The listing builds one solid part. Answer for the finished solid, in the listing's coordinates (mm). Give positions to 0.01 mm unless a question says otherwise; leave off trailing zeros. Order: outer loops, then holes, each group sorted by start corner. A loop starts at its lowest first (then second) coordinate and runs counter-clockwise, first axis right, second up. Notation, with made-up numbers: (63.25, 51) - (88.25, 51) arc R15 ccw to (88.25, 76) - close; hole circle Ø5 at (-35.75, -35). An arc over 180 degrees is marked (long way). Use CSV: the item, a comma, the result in double quotes.
```python
from build123d import *

# Parameters (mm, degrees)
F0_R     = 7
F0_R_2   = 1.55
F1_DEPTH = 7
F2_R     = 1
F3_R     = 4
F4_DEPTH = 3


with BuildPart() as f1:
    # F0 (on Front) → F1 (new body)
    with BuildSketch(Plane.XZ):
        with Locations((-31.374283, 43.221928)):
            Circle(F0_R)
        with Locations((-31.374283, 43.221928)):
            Circle(F0_R_2, mode=Mode.SUBTRACT)
    extrude(amount=F1_DEPTH)

    # F2
    f2_edges = [f1.edges().sort_by_distance(p)[0] for p in [
        (-38.374283, -7, 43.221928),
    ]]
    fillet(f2_edges, radius=F2_R)

    # F3 (on face) → F4 (cut)
    with BuildSketch(Plane.XZ.offset(7)):
        with Locations((-31.374283, 43.221928)):
            Circle(F3_R)
    extrude(amount=-F4_DEPTH, mode=Mode.SUBTRACT)


solid = f1.part
```
Item 1: Each of these flat-tipped pins is pushed along its axis until it touches: pin 1 (1 mm diameter, centred on x = -30.5, y = -3.5, fed in from +Z); pin 2 (2.5 mm diameter, centred on x = -33, z = 45, fed in from -Y); pin 3 (3 mm diameter, centred on x = -26.5, y = -4, fed in from +Z) (3 decimals). Where does it stop, or does it pass through?
Taken from the geometry:
pin 1,"z = 50.21"
pin 2,"y = -4"
pin 3,"z = 49.355"
Item 2: The part is cut by section A-A (y = -1.75). Give the vertices of the cut face in (x, z), and give its area (3 significant figures).
Taken from the geometry:
outline,"circle Ø14 at (-31.37, 43.22); hole circle Ø3.1 at (-31.37, 43.22)"
area,"146 mm^2"
Item 3: The part is cut by section B-B (y = -5.75). Give the vertices of the cut face in (x, z).
Taken from the geometry:
outline,"circle Ø14 at (-31.37, 43.22); hole circle Ø8 at (-31.37, 43.22)"
Item 4: Find the intervals of material crossed by line 1 along Z through (x, y) = (-31.5, -4.5); line 2 along Y through (x, z) = (-32.5, 40); line 3 along X through (y, z) = (-2.25, 44), in increasing order.
Taken from the geometry:
line 1,"36.22 to 39.22, 47.22 to 50.22"
line 2,"-4 to 0"
line 3,"-38.33 to -32.71, -30.03 to -24.42"
Item 5: The mould has two halves that part along Z. Classify faces 1 (the face through (-34.32, -5.52, 45.93)), 2 (the face through (-38.368, -2.958, 43.53)), 3 (the face through (-30, -7, 39)), 4 (the face through (-31.4, -4, 41.5)): +Z half, -Z half, draft (parallel to the pull), parting line (faces both ways), or undercut.
Taken from the geometry:
face 1,"undercut"
face 2,"parting line"
face 3,"draft"
face 4,"undercut"
